Read the model definition and answer for the solid it produces. Units are mm, in the model's axes. Face numbers are marked on the shaded views. Give positions to 0.01 mm unless a question says otherwise; leave off trailing zeros. Loops run counter-clockwise (first coordinate to the right, second up) from the corner with the lowest first, then second, coordinate; pieces in that order, holes last. Notation, with made-up numbers: (83.5, -34.75) -> (117.5, -34.75) arc R37 cw to (117.5, 2.25) -> close; hole circle Ø8 at (57.5, 48). An arc over 180 degrees is marked (long way). Answer as CSV lines item,"result". Start each with the question number.
```python
from build123d import *

# Parameters (mm, degrees)
F1_DEPTH = 18.25625
F2_W     = 457.2
F2_H     = 38.1
F3_DEPTH = 88.9
F4_R     = 25.4
F5_R     = 6.35


with BuildPart() as f1:
    # F0 (on Right) → F1 (new body)
    with BuildSketch(Plane.YZ):
        with BuildLine():
            Line((0, 1422.4), (0, 0))
            Line((0, 0), (1041.4, 0))
            Line((1041.4, 0), (1041.4, 1422.4))
            ThreePointArc((1041.4, 1422.4), (1033.960512, 1440.360512), (1016, 1447.8))
            Line((1016, 1447.8), (769.675159, 1447.8))
            ThreePointArc((769.675159, 1447.8), (753.781683, 1442.213062), (744.880007, 1427.910034))
            Line((744.880007, 1427.910034), (702.919993, 1239.089966))
            ThreePointArc((702.919993, 1239.089966), (694.018317, 1224.786938), (678.124841, 1219.2))
            Line((678.124841, 1219.2), (363.275159, 1219.2))
            ThreePointArc((363.275159, 1219.2), (347.381683, 1224.786938), (338.480007, 1239.089966))
            Line((338.480007, 1239.089966), (296.519993, 1427.910034))
            ThreePointArc((296.519993, 1427.910034), (287.618317, 1442.213062), (271.724841, 1447.8))
            Line((271.724841, 1447.8), (25.4, 1447.8))
            ThreePointArc((25.4, 1447.8), (7.439488, 1440.360512), (0, 1422.4))
        make_face()
    extrude(amount=F1_DEPTH)

    # F2 (on face) → F3 (join)
    with BuildSketch(Plane.YZ.offset(18.25625)):
        with Locations((520.7, 209.55)):
            Rectangle(F2_W, F2_H)
        with Locations((520.7, 438.15)):
            Rectangle(F2_W, F2_H)
        with Locations((520.7, 666.75)):
            Rectangle(F2_W, F2_H)
        with Locations((520.7, 895.35)):
            Rectangle(F2_W, F2_H)
    extrude(amount=F3_DEPTH)

    # F4
    f4_edges = [f1.edges().sort_by_distance(p)[0] for p in [
        (107.15625, 292.1, 895.35),
        (107.15625, 749.3, 895.35),
        (107.15625, 292.1, 666.75),
        (107.15625, 749.3, 666.75),
        (107.15625, 292.1, 438.15),
        (107.15625, 292.1, 209.55),
        (107.15625, 749.3, 209.55),
    ]]
    fillet(f4_edges, radius=F4_R)

    # F5
    f5_edges = [f1.edges().sort_by_distance(p)[0] for p in [
        (50.00625, 292.1, 914.4),
        (50.00625, 292.1, 876.3),
        (50.00625, 292.1, 685.8),
        (50.00625, 292.1, 647.7),
        (50.00625, 292.1, 457.2),
        (50.00625, 292.1, 419.1),
        (50.00625, 292.1, 228.6),
        (50.00625, 292.1, 190.5),
    ]]
    fillet(f5_edges, radius=F5_R)


solid = f1.part
```
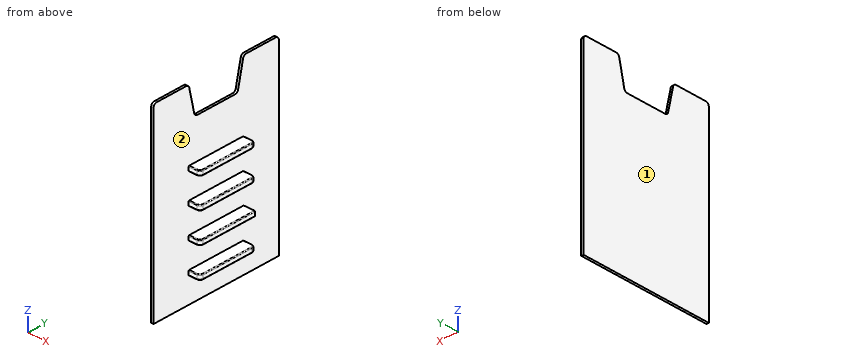
(1) Find section C-C on z = 1178.5. Write down the section's boundary in (x, y).
(2) Find section B-B on y = 487.5. Write down the section's boundary in (x, z).
(3) Each of these flat-tipped pins is pushed along its axis until it touches: P1, Ø5, axis at x = 93.5, y = 308, coming from the +Z side; P2, Ø12, axis at x = 59.5, y = 681, coming from the -Z side; P3, Ø12.5, axis at x = 45, z = 664.5, coming from the -Y side. Where does it stop, or does it pass through?
(4) Find the intervals of material crossed by line 1 along Z through (x, y) = (56, 324); line 2 along X through (y, z) = (833, 1069), in increasing order. Write a range as from..to.
(5) Find section D-D on y = 946.5. Write down the section's boundary in (x, z), then the cut area to 3 significant figures.
(6) Find section A-A on x = 48. Give the number of separate pieces and of enclosed holes in the cut face, then the cut area to 3 significant figures.
(7) The mould has two halves that part along Z. Classify the marked faces 1 and 2: pulls with the +Z half, pulls with the -Z half, needs draft (parallel to the pull), parting line crosses it, or undercut.
Answer block:
1,outline,"(0, 0) -> (18.26, 0) -> (18.26, 1041.4) -> (0, 1041.4) -> close"
2,outline,"(0, 0) -> (18.26, 0) -> (18.26, 190.5) -> (100.81, 190.5) arc R6.35 ccw to (107.16, 196.85) -> (107.16, 222.25) arc R6.35 ccw to (100.81, 228.6) -> (18.26, 228.6) -> (18.26, 419.1) -> (100.81, 419.1) arc R6.35 ccw to (107.16, 425.45) -> (107.16, 450.85) arc R6.35 ccw to (100.81, 457.2) -> (18.26, 457.2) -> (18.26, 647.7) -> (100.81, 647.7) arc R6.35 ccw to (107.16, 654.05) -> (107.16, 679.45) arc R6.35 ccw to (100.81, 685.8) -> (18.26, 685.8) -> (18.26, 876.3) -> (100.81, 876.3) arc R6.35 ccw to (107.16, 882.65) -> (107.16, 908.05) arc R6.35 ccw to (100.81, 914.4) -> (18.26, 914.4) -> (18.26, 1219.2) -> (0, 1219.2) -> close"
3,P1,"stops at z = 914.4"
3,P2,"stops at z = 190.5"
3,P3,"stops at y = 292.1"
4,line 1,"z = 190.5..228.6, 419.1..457.2, 647.7..685.8, 876.3..914.4"
4,line 2,"x = 0..18.26"
5,outline,"(0, 0) -> (18.26, 0) -> (18.26, 1447.8) -> (0, 1447.8) -> close"
5,area,"26,400 mm2"
6,separate pieces,"4"
6,enclosed holes,"0"
6,area,"69,600 mm2"
7,face 1,"needs draft"
7,face 2,"undercut"
